Build history of the part. All positions in model axes, mm. Face numbers are marked on the shaded views. A direction names the side the tool comes from. Give positions to 0.01 mm unless a question says otherwise; leave off trailing zeros. Write each loop counter-clockwise with the first axis right and the second up, starting at its lowest first coordinate (ties: lowest second). Pieces come first, ordered by that corner, then holes. Notation, with made-up numbers: (32.5, 61) -> (73.5, 61) arc R20 ccw to (73.5, 99) -> close; hole circle Ø5 at (-35.75, -37.5). An arc over 180 degrees is marked (long way). One line per question, with ' | ' between items. Start each with the question number.
(1) Band-saw the part on A-A, the plane z = 0. Give the cut face in (x, y).
(2) Pin check, flat tips, straight feed: P1, Ø1.9, axis at y = 8.5, z = -19, coming from the +X side; P2, Ø1.9, axis at x = -18.5, y = 6, coming from the -Z side; P3, Ø0.8, axis at x = 1, z = -19, coming from the +Y side; P4, Ø2, axis at x = -10, z = 1, coming from the -Y side. Stop position of each tip, or through.
(3) Drill centre lines: probe 1 along Z at (x, y) = (12.5, 4.5); probe 2 along X at (y, z) = (9, -11.5); probe 3 along X at (y, z) = (7, -10.5). Where is each one in solid material? Low to high. Write a range as from..to.
(4) Band-saw the part on B-B, the plane x = 16. Give the cut face in (y, z), and give its area (3 significant figures).
(5) Pull direction Z, two halves, no side cores. Call the marked faces 1, 2, 3 and 4: released by +Z, released by -Z, zero draft, split by the parting line, or undercut.
(6) Tool access for the marked faces 5 and 6: list every direction of +Z, -Z, +X, -X, +Y, -Y with a clear straight run to the whole face (end or side of a thin tool).
(7) Band-saw the part on D-D, the plane y = 5.25. Count the separate pieces of the cut face and the enclosed holes in it, and give its area (3 significant figures).
(8) Band-saw the part on C-C, the plane x = 0. Give the cut face in (y, z).
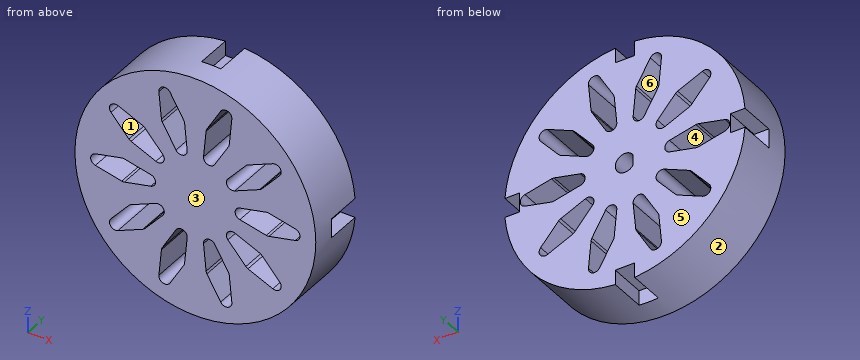
from build123d import *

# Parameters (mm, degrees)
SKETCH_1_R               = 20
SKETCH_1_R_2             = 4
EXTRUDE_1_DEPTH          = 10
SKETCH_4_R               = 20
EXTRUDE_2_DEPTH          = 6
SKETCH_5_R               = 1.6
CUT_EXTRUDE_2_DEPTH      = 5
CUT_EXTRUDE_2_DEPTH_BACK = 7
CUT_EXTRUDE_3_DEPTH      = 1
CUT_EXTRUDE_3_DEPTH_BACK = 11
SKETCH_8_W               = 3.2
SKETCH_8_H               = 5
SKETCH_8_W_2             = 5
SKETCH_8_H_2             = 3.2
CUT_EXTRUDE_4_DEPTH      = 6
SKETCH_9_R               = 3
CUT_EXTRUDE_5_DEPTH      = 2
SKETCH_11_R              = 4
EXTRUDE_3_DEPTH          = 4
SKETCH_12_R              = 3
EXTRUDE_4_DEPTH          = 2
SKETCH_13_R              = 1.6
EXTRUDE_5_DEPTH          = 2


with BuildPart() as part:
    # Эскиз1 → Бобышка-Вытянуть1 (new body)
    with BuildSketch(Plane(origin=(0, 0, 0), x_dir=(1, 0, 0), z_dir=(0, 1, 0))):
        Circle(SKETCH_1_R)
        Circle(SKETCH_1_R_2, mode=Mode.SUBTRACT)
    extrude(amount=EXTRUDE_1_DEPTH)

    # Эскиз4 → Бобышка-Вытянуть2 (add)
    with BuildSketch(Plane.XZ):
        Circle(SKETCH_4_R)
    extrude(amount=-EXTRUDE_2_DEPTH)

    # Эскиз5 → Вырез-Вытянуть2 (cut, two sides)
    with BuildSketch(Plane(origin=(0, 6, 0), x_dir=(1, 0, 0), z_dir=(0, 1, 0))) as cut_extrude_2_sk:
        Circle(SKETCH_5_R)
    extrude(amount=CUT_EXTRUDE_2_DEPTH, mode=Mode.SUBTRACT)
    extrude(cut_extrude_2_sk.sketch, amount=-CUT_EXTRUDE_2_DEPTH_BACK, mode=Mode.SUBTRACT)

    # Эскиз6 → Вырез-Вытянуть3 (cut, two sides)
    with BuildSketch(Plane.XZ) as cut_extrude_3_sk:
        with BuildLine():
            Line((-7.392842, 0.976187), (-11.78307, 1.951793))
            ThreePointArc((-11.78307, 1.951793), (-12, 1.975606), (-12.21693, 1.951793))
            Line((-12.21693, 1.951793), (-16.607158, 0.976187))
            ThreePointArc((-16.607158, 0.976187), (-17.390228, 0), (-16.607158, -0.976187))
            Line((-16.607158, -0.976187), (-12.21693, -1.951793))
            ThreePointArc((-12.21693, -1.951793), (-12, -1.975606), (-11.78307, -1.951793))
            Line((-11.78307, -1.951793), (-7.392842, -0.976187))
            ThreePointArc((-7.392842, -0.976187), (-6.609772, 0), (-7.392842, 0.976187))
        make_face()
        with BuildLine():
            Line((-5.407146, 5.135155), (-8.385468, 8.504948))
            ThreePointArc((-8.385468, 8.504948), (-8.546972, 8.651722), (-8.736469, 8.759965))
            Line((-8.736469, 8.759965), (-12.861685, 10.551195))
            ThreePointArc((-12.861685, 10.551195), (-14.06899, 10.221719), (-14.009262, 8.971691))
            Line((-14.009262, 8.971691), (-11.03094, 5.601898))
            ThreePointArc((-11.03094, 5.601898), (-10.869436, 5.455124), (-10.679939, 5.346881))
            Line((-10.679939, 5.346881), (-6.554723, 3.555651))
            ThreePointArc((-6.554723, 3.555651), (-5.347418, 3.885127), (-5.407146, 5.135155))
        make_face()
        with BuildLine():
            Line((-1.356105, 7.332669), (-1.784903, 11.809502))
            ThreePointArc((-1.784903, 11.809502), (-1.829291, 12.023174), (-1.918973, 12.222129))
            Line((-1.918973, 12.222129), (-4.203485, 16.096004))
            ThreePointArc((-4.203485, 16.096004), (-5.373876, 16.539089), (-6.060303, 15.492688))
            Line((-6.060303, 15.492688), (-5.631505, 11.015854))
            ThreePointArc((-5.631505, 11.015854), (-5.587117, 10.802182), (-5.497434, 10.603228))
            Line((-5.497434, 10.603228), (-3.212923, 6.729352))
            ThreePointArc((-3.212923, 6.729352), (-2.042532, 6.286267), (-1.356105, 7.332669))
        make_face()
        with BuildLine():
            Line((3.212923, 6.729352), (5.497434, 10.603228))
            ThreePointArc((5.497434, 10.603228), (5.587117, 10.802182), (5.631505, 11.015854))
            Line((5.631505, 11.015854), (6.060303, 15.492688))
            ThreePointArc((6.060303, 15.492688), (5.373876, 16.539089), (4.203485, 16.096004))
            Line((4.203485, 16.096004), (1.918973, 12.222129))
            ThreePointArc((1.918973, 12.222129), (1.829291, 12.023174), (1.784903, 11.809502))
            Line((1.784903, 11.809502), (1.356105, 7.332669))
            ThreePointArc((1.356105, 7.332669), (2.042532, 6.286267), (3.212923, 6.729352))
        make_face()
        with BuildLine():
            Line((6.554723, 3.555651), (10.679939, 5.346881))
            ThreePointArc((10.679939, 5.346881), (10.869436, 5.455124), (11.03094, 5.601898))
            Line((11.03094, 5.601898), (14.009262, 8.971691))
            ThreePointArc((14.009262, 8.971691), (14.06899, 10.221719), (12.861685, 10.551195))
            Line((12.861685, 10.551195), (8.736469, 8.759965))
            ThreePointArc((8.736469, 8.759965), (8.546972, 8.651722), (8.385468, 8.504948))
            Line((8.385468, 8.504948), (5.407146, 5.135155))
            ThreePointArc((5.407146, 5.135155), (5.347418, 3.885127), (6.554723, 3.555651))
        make_face()
        with BuildLine():
            Line((7.392842, -0.976187), (11.78307, -1.951793))
            ThreePointArc((11.78307, -1.951793), (12, -1.975606), (12.21693, -1.951793))
            Line((12.21693, -1.951793), (16.607158, -0.976187))
            ThreePointArc((16.607158, -0.976187), (17.390228, 0), (16.607158, 0.976187))
            Line((16.607158, 0.976187), (12.21693, 1.951793))
            ThreePointArc((12.21693, 1.951793), (12, 1.975606), (11.78307, 1.951793))
            Line((11.78307, 1.951793), (7.392842, 0.976187))
            ThreePointArc((7.392842, 0.976187), (6.609772, 0), (7.392842, -0.976187))
        make_face()
        with BuildLine():
            Line((5.407146, -5.135155), (8.385468, -8.504948))
            ThreePointArc((8.385468, -8.504948), (8.546972, -8.651722), (8.736469, -8.759965))
            Line((8.736469, -8.759965), (12.861685, -10.551195))
            ThreePointArc((12.861685, -10.551195), (14.06899, -10.221719), (14.009262, -8.971691))
            Line((14.009262, -8.971691), (11.03094, -5.601898))
            ThreePointArc((11.03094, -5.601898), (10.869436, -5.455124), (10.679939, -5.346881))
            Line((10.679939, -5.346881), (6.554723, -3.555651))
            ThreePointArc((6.554723, -3.555651), (5.347418, -3.885127), (5.407146, -5.135155))
        make_face()
        with BuildLine():
            Line((1.356105, -7.332669), (1.784903, -11.809502))
            ThreePointArc((1.784903, -11.809502), (1.829291, -12.023174), (1.918973, -12.222129))
            Line((1.918973, -12.222129), (4.203485, -16.096004))
            ThreePointArc((4.203485, -16.096004), (5.373876, -16.539089), (6.060303, -15.492688))
            Line((6.060303, -15.492688), (5.631505, -11.015854))
            ThreePointArc((5.631505, -11.015854), (5.587117, -10.802182), (5.497434, -10.603228))
            Line((5.497434, -10.603228), (3.212923, -6.729352))
            ThreePointArc((3.212923, -6.729352), (2.042532, -6.286267), (1.356105, -7.332669))
        make_face()
        with BuildLine():
            Line((-3.212923, -6.729352), (-5.497434, -10.603228))
            ThreePointArc((-5.497434, -10.603228), (-5.587117, -10.802182), (-5.631505, -11.015854))
            Line((-5.631505, -11.015854), (-6.060303, -15.492688))
            ThreePointArc((-6.060303, -15.492688), (-5.373876, -16.539089), (-4.203485, -16.096004))
            Line((-4.203485, -16.096004), (-1.918973, -12.222129))
            ThreePointArc((-1.918973, -12.222129), (-1.829291, -12.023174), (-1.784903, -11.809502))
            Line((-1.784903, -11.809502), (-1.356105, -7.332669))
            ThreePointArc((-1.356105, -7.332669), (-2.042532, -6.286267), (-3.212923, -6.729352))
        make_face()
        with BuildLine():
            Line((-6.554723, -3.555651), (-10.679939, -5.346881))
            ThreePointArc((-10.679939, -5.346881), (-10.869436, -5.455124), (-11.03094, -5.601898))
            Line((-11.03094, -5.601898), (-14.009262, -8.971691))
            ThreePointArc((-14.009262, -8.971691), (-14.06899, -10.221719), (-12.861685, -10.551195))
            Line((-12.861685, -10.551195), (-8.736469, -8.759965))
            ThreePointArc((-8.736469, -8.759965), (-8.546972, -8.651722), (-8.385468, -8.504948))
            Line((-8.385468, -8.504948), (-5.407146, -5.135155))
            ThreePointArc((-5.407146, -5.135155), (-5.347418, -3.885127), (-6.554723, -3.555651))
        make_face()
    extrude(amount=CUT_EXTRUDE_3_DEPTH, mode=Mode.SUBTRACT)
    extrude(cut_extrude_3_sk.sketch, amount=-CUT_EXTRUDE_3_DEPTH_BACK, mode=Mode.SUBTRACT)

    # Эскиз8 → Вырез-Вытянуть4 (cut)
    with BuildSketch(Plane(origin=(0, 10, 0), x_dir=(1, 0, 0), z_dir=(0, 1, 0))):
        with Locations((0, 20)):
            Rectangle(SKETCH_8_W, SKETCH_8_H)
        with Locations((-20, 0)):
            Rectangle(SKETCH_8_W_2, SKETCH_8_H_2)
        with Locations((20, 0)):
            Rectangle(SKETCH_8_W_2, SKETCH_8_H_2)
        with Locations((0, -20)):
            Rectangle(SKETCH_8_W, SKETCH_8_H)
    extrude(amount=-CUT_EXTRUDE_4_DEPTH, mode=Mode.SUBTRACT)

    # Эскиз9 → Вырез-Вытянуть5 (cut)
    with BuildSketch(Plane.XZ):
        Circle(SKETCH_9_R)
    extrude(amount=-CUT_EXTRUDE_5_DEPTH, mode=Mode.SUBTRACT)

    # Эскиз11 → Бобышка-Вытянуть3 (add)
    with BuildSketch(Plane(origin=(0, 6, 0), x_dir=(1, 0, 0), z_dir=(0, 1, 0))):
        Circle(SKETCH_11_R)
        with BuildLine():
            Line((-1.3, 0.932738), (-1.3, -0.932738))
            ThreePointArc((-1.3, -0.932738), (1.6, 0), (-1.3, 0.932738))
        make_face(mode=Mode.SUBTRACT)
    extrude(amount=EXTRUDE_3_DEPTH)

    # Эскиз12 → Бобышка-Вытянуть4 (add)
    with BuildSketch(Plane.XZ.offset(-2)):
        Circle(SKETCH_12_R)
    extrude(amount=EXTRUDE_4_DEPTH)

    # Эскиз13 → Бобышка-Вытянуть5 (add)
    with BuildSketch(Plane(origin=(0, 2, 0), x_dir=(1, 0, 0), z_dir=(0, 1, 0))):
        Circle(SKETCH_13_R)
    extrude(amount=EXTRUDE_5_DEPTH)


solid = part.part
Results:
1) outline: (-20, 0) -> (-17.39, 0) -> (-17.39, 10) -> (-17.5, 10) -> (-17.5, 4) -> (-20, 4) -> close; (-6.61, 0) -> (6.61, 0) -> (6.61, 10) -> (1.6, 10) -> (1.6, 4) -> (-1.6, 4) -> (-1.6, 6) -> (-1.3, 6) -> (-1.3, 10) -> (-6.61, 10) -> close; (17.39, 0) -> (20, 0) -> (20, 4) -> (17.5, 4) -> (17.5, 10) -> (17.39, 10) -> close
2) P1: stops at x = 8.61 | P2: stops at z = -9.59 | P3: stops at y = 4 | P4: stops at y = 0
3) probe 1: z = -15.61..-10.39, -7.26..-1.89, 1.89..7.26, 10.39..15.61 | probe 2: x = -16.36..-5.68, -1.76..1.76, 5.68..16.36 | probe 3: x = -17.02..-13.76, -12.74..-5.44, -1.66..1.66, 5.44..12.74, 13.76..17.02
4) outline: (0, -12) -> (10, -12) -> (10, -1.11) -> (0, -1.11) -> close; (0, 1.11) -> (10, 1.11) -> (10, 12) -> (0, 12) -> close | area: 218 mm²
5) face 1: undercut | face 2: split by the parting line | face 3: zero draft | face 4: undercut
6) face 5: +Z, -Z, +X, -X, +Y | face 6: +Y, -Y
7) separate pieces: 1 | enclosed holes: 11 | area: 920 mm²
8) outline: (0, -20) -> (4, -20) -> (4, -17.5) -> (10, -17.5) -> (10, -1.6) -> (4, -1.6) -> (4, 1.6) -> (10, 1.6) -> (10, 17.5) -> (4, 17.5) -> (4, 20) -> (0, 20) -> close
